from build123d import *

# Parameters (mm, degrees)
EXTRUDE_1_DEPTH = 3


with BuildPart() as part:
    # 草图1 → 凸台-拉伸1 (new body)
    with BuildSketch(Plane.XY):
        with BuildLine():
            ThreePointArc((6, 0), (7.5, 1.5), (9, 0))
            Line((9, 0), (15, 0))
            ThreePointArc((15, 0), (7.5, 7.5), (0, 0))
            Line((0, 0), (6, 0))
        make_face()
        with BuildLine():
            ThreePointArc((9, 0), (8.560660172, -1.060660172), (7.5, -1.5))
            Line((7.5, -1.5), (7.5, -7.5))
            ThreePointArc((7.5, -7.5), (12.803300859, -5.303300859), (15, 0))
            Line((15, 0), (9, 0))
        make_face()
        with BuildLine():
            Line((7.5, -7.5), (7.5, -1.5))
            ThreePointArc((7.5, -1.5), (6.439339828, -1.060660172), (6, 0))
            Line((6, 0), (0, 0))
            ThreePointArc((0, 0), (2.196699141, -5.303300859), (7.5, -7.5))
        make_face()
        with BuildLine():
            ThreePointArc((15, 0), (12.803300859, -5.303300859), (7.5, -7.5))
            Line((7.5, -7.5), (7.5, -22))
            Line((7.5, -22), (12.5, -22))
            Line((12.5, -22), (15, -22))
            Line((15, -22), (15, 0))
        make_face()
        with BuildLine():
            Line((7.5, -22), (7.5, -7.5))
            ThreePointArc((7.5, -7.5), (2.196699141, -5.303300859), (0, 0))
            Line((0, 0), (0, -22))
            Line((0, -22), (2.5, -22))
            Line((2.5, -22), (7.5, -22))
        make_face()
        Polygon((12.5, -22), (7.5, -22), (2.5, -22), (2.5, -25), (12.5, -25), align=None)
    extrude(amount=EXTRUDE_1_DEPTH)


solid = part.part
Geometry: final body of the model. Coordinates: model frame, mm. A direction names the side the tool comes from. Coordinates: 2 decimals unless noted, no trailing zeros. Loops run counter-clockwise (first coordinate to the right, second up) from the corner with the lowest first, then second, coordinate; pieces in that order, holes last. Notation, with made-up numbers: M -20,-4.5 L -10,-4.5 A23 ccw -10,15.5 Z; hole C -21.75,-23 d6. An arc over 180 degrees is marked long. One line per item, written item: value. Start each with the question number.
1) Cut plane C-C (x = 6.75). Return loops of the section in (y, z).
2) Cut plane B-B (z = 2.5). Return loops of the section in (x, y), then the cut area to 3 significant figures.
3) Cut plane A-A (y = -1). Return loops of the section in (x, z).
4) Material intervals for L1, parallel to Y at x = 3, z = 1.7; L2, parallel to X at y = -1, z = 1.05; L3, parallel to X at y = -0.5, z = 2.45, sorted ascending. Write a range as from..to.
5) Cut plane D-D (x = 13.5). Return loops of the section in (y, z), then the cut area to 3 significant figures.
6) Pin query (flat end, axial travel): P1, Ø1, axis at x = 4, z = 2.5, coming from the +Y side. Return the tip coordinate at first contact, or that it passes through.
7) Reachability of faces 1 (the flat face through (15, -11, 1)), 2 (the flat face through (1, -22, 1)), 3 (the flat face through (12.5, -24, 1)) from +Z, -Z, +X, -X, +Y, -Y: full face, straight path, thin tool, end or side. Return the list, or none.
Evaluation:
1. outline: M -25,0 L -1.3,0 L -1.3,3 L -25,3 Z; M 1.3,0 L 7.46,0 L 7.46,3 L 1.3,3 Z
2. outline: M 0,-22 L 2.5,-22 L 2.5,-25 L 12.5,-25 L 12.5,-22 L 15,-22 L 15,0 A7.5 ccw 0,0 Z; hole C 7.5,0 d3
2. area: 441 mm^2
3. outline: M 0,0 L 6.38,0 L 6.38,3 L 0,3 Z; M 8.62,0 L 15,0 L 15,3 L 8.62,3 Z
4. L1: -25..6
4. L2: 0..6.38, 8.62..15
4. L3: 0..6.09, 8.91..15
5. outline: M -22,0 L 4.5,0 L 4.5,3 L -22,3 Z
5. area: 79.5 mm^2
6. P1: y = 6.87
7. face 1: +Z, -Z, +X, +Y, -Y
7. face 2: +Z, -Z, -X, -Y
7. face 3: +Z, -Z, +X, -Y
